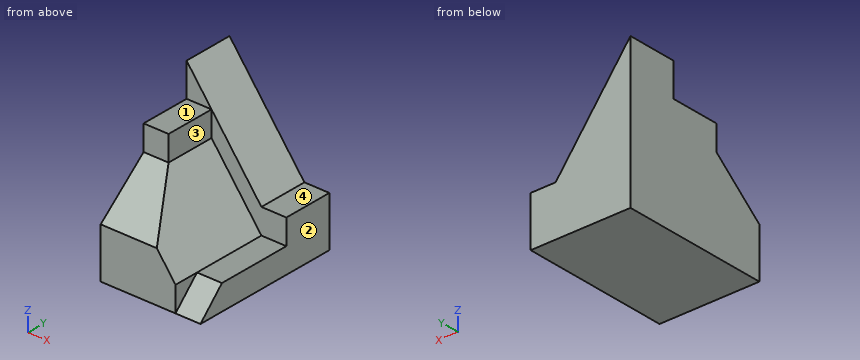
```python
from build123d import *

# Parameters (mm, degrees)
F1_DEPTH = 30
F3_DEPTH = 20
F5_DEPTH = 20.001
F7_DEPTH = 5


with BuildPart() as f1:
    # F0 (on Front) → F1 (new body)
    with BuildSketch(Plane.XZ):
        Polygon((0, 30), (0, 0), (20, 0), (20, 10), (15, 10), align=None)
    extrude(amount=-F1_DEPTH)

    # F2 (on face) → F3 (cut)
    with BuildSketch(Plane.XZ):
        Polygon((0, 30), (0, 23.3333333333), (5, 23.3333333333), align=None)
        Polygon((15, 10), (5, 23.3333333333), (5, 18.3333333333), (15, 5), (20, 5), (20, 10), align=None)
    extrude(amount=-F3_DEPTH, mode=Mode.SUBTRACT)

    # F4 (on face) → F5 (cut, through all)
    with BuildSketch(Plane(origin=(0, 0, 0), x_dir=(0, -1, 0), z_dir=(-1, 0, 0))):
        Polygon((0, 23.3333333333), (-10, 23.3333333333), (-10, 18.3333333333), (0, 10), align=None)
    extrude(amount=-F5_DEPTH, mode=Mode.SUBTRACT)

    # F6 (on face) → F7 (cut, through all)
    with BuildSketch(Plane.YZ.offset(20)):
        Polygon((0, 5), (0, 0), (5, 5), align=None)
    extrude(amount=-F7_DEPTH, mode=Mode.SUBTRACT)


solid = f1.part
```
Source: CAD feature listing. Evaluate the final solid. Frame: model axes, mm. Face numbers are marked on the shaded views. A direction names the side the tool comes from. Round coordinates to 2 decimals unless told otherwise and drop trailing zeros. Loops run counter-clockwise (first coordinate to the right, second up) from the corner with the lowest first, then second, coordinate; pieces in that order, holes last. Notation, with made-up numbers: M -36.75,-6 L 9.25,-6 A15 ccw 9.25,0 Z; hole C 79.5,-18.75 d9. An arc over 180 degrees is marked long. Use a Markdown table: item, result. Add a question column.
1. Cut plane C-C, the plane x = 7.5. Output: boundary loops of the cut face in (y, z).
2. Cut plane A-A, the plane y = 14.25. Output: boundary loops of the cut face in (x, z).
3. Contact query for flat-ended pins moving along their axis: pin 1 (1 mm diameter, centred on x = 2.5, y = 8, fed in from -Z); pin 2 (4 mm diameter, centred on x = 18.5, y = 10, fed in from +Z); pin 3 (7.5 mm diameter, centred on x = 15, z = 13.5, fed in from -Y); pin 4 (5 mm diameter, centred on x = 2.5, z = 21.5, fed in from -Y). Output: stop coordinate, or through.
4. Ray query, line 1 along Z through (x, y) = (17, 15); line 2 along Y through (x, z) = (19, 8.25); line 3 along Z through (x, y) = (15.75, 22.25). Return the intervals inside material, ascending. Write a range as [from, to].
5. Cut plane B-B, the plane z = 17. Output: boundary loops of the cut face in (x, y), and give its area (3 significant figures).
6. Set-up query: the marked faces 1, 2, 3 and 4. Return all of +Z, -Z, +X, -X, +Y, -Y with unobstructed straight access to the full face (end or side cutting, diameter ignored); none if empty.
7. Cut plane D-D, the plane y = 21.5. Output: boundary loops of the cut face in (x, z).
Solution:
| question | item | result |
|---|---|---|
| 1 | outline | M 0,0 L 30,0 L 30,20 L 20,20 L 20,15 L 6,15 L 0,10 Z |
| 2 | outline | M 0,0 L 20,0 L 20,5 L 15,5 L 5,18.33 L 5,23.33 L 0,23.33 Z |
| 3 | pin 1 | stops at z = 0 |
| 3 | pin 2 | stops at z = 5 |
| 3 | pin 3 | stops at y = 20 |
| 3 | pin 4 | stops at y = 10 |
| 4 | line 1 | z = [0, 5] |
| 4 | line 2 | y = [20, 30] |
| 4 | line 3 | z = [0, 10] |
| 5 | outline | M 0,8.4 L 6,8.4 L 6,20 L 9.75,20 L 9.75,30 L 0,30 Z |
| 5 | area | 167 mm2 |
| 6 | face 1 | +Z, +X, -X, -Y |
| 6 | face 2 | +Z, -Z, +X, +Y, -Y |
| 6 | face 3 | +Z, +X, -Y |
| 6 | face 4 | +Z, +X, +Y, -Y |
| 7 | outline | M 0,0 L 20,0 L 20,10 L 15,10 L 0,30 Z |
